Geometry check sheet. Reference: the model listing, model coordinates, mm. A direction names the side the tool comes from. Round coordinates to 2 decimals unless told otherwise and drop trailing zeros. Order: outer loops, then holes, each group sorted by start corner. A loop starts at its lowest first (then second) coordinate and runs counter-clockwise, first axis right, second up.
(1) Sectioned sample at B-B (z = -223.5). Record the boundary of the cut face in (x, y), plus the area to 3 significant figures.
(2) Material ranges on line 1 along Z through (x, y) = (-279.5, 146.5); line 2 along Y through (x, z) = (-217, -430); line 3 along Z through (x, y) = (-248.5, 277.5), recorded low to high.
(3) Release check for a two-part mould opening along Z. For faces 4 (the face through (-254, 218, -240)), 5 (the face through (-301, 225, -225)), 6 (the face through (-305.51, 182.74, -204.18)) record: +Z half, -Z half, draft (parallel to the pull), parting line (faces both ways), or undercut.
(4) Sectioned sample at C-C (x = -242). Record the boundary of the cut face in (y, z) (3 decimals).
(5) Sectioned sample at A-A (y = 182.5). Record the boundary of the cut face in (x, z).
(6) Go/stop test with flat-tipped pins: pin 1 (4 mm diameter, centred on x = -132.5, z = -308.5, fed in from -Y); pin 2 (6 mm diameter, centred on x = -491, y = 325, fed in from +Z); pin 3 (6 mm diameter, centred on x = -537.5, z = -295.5, fed in from -Y). Record where each tip stops, or that it passes through.
(7) Sectioned sample at D-D (y = 88). Record the boundary of the cut face in (x, z), plus the area to 3 significant figures.
(8) Set-up check for faces 1 (the face through (-304.089, 254.483, -276.121)), 2 (the face through (-305.511, 208.996, -248.735)), 3 (the face through (-355.6, 219, -241)): record each of +Z, -Z, +X, -X, +Y, -Y from which the full face is reachable in a straight line by a thin tool's end or side.
Autodesk Inventor part; units mm, degrees
ref_plane "YZ Plane" through (0, 0, 0) normal (1, 0, 0) x (0, 1, 0)
ref_plane "XZ Plane" through (0, 0, 0) normal (0, 1, 0) x (-1, 0, 0)
ref_plane "XY Plane" through (0, 0, 0) normal (0, 0, 1) x (1, 0, 0)
sketch "Sketch6" plane through (0, 0, 0) normal (0, 1, 0) x (-1, 0, 0)
  line L0 (0, 0) -> (609.6, 0)
  line L1 (609.6, 0) -> (609.6, -914.4)
  line L2 (609.6, -914.4) -> (0, -914.4)
  line L3 (0, -914.4) -> (0, 0)
  dimension "d21" = 609.6
  dimension "d22" = 914.4
extrude "Extrusion6" add sketch "Sketch6" along normal blind 609.6
sketch "Sketch8" plane through (0, 0, 0) normal (1, 0, 0) x (0, 0, -1)
  line L0 (0, 609.6) -> (914.4, 609.6)
  line L1 (0, 0) -> (457.2, 0) construction
  line L2 (0, 0) -> (457.2, 457.2)
  line L3 (0, 0) -> (646.5784, 0) construction
  line L4 (457.2, 457.2) -> (914.4, 0)
  line L5 (457.2, 457.2) -> (459.4451, 454.9549)
  line L6 (0, 0) -> (3.175, 0)
  line L7 (3.175, 0) -> (459.4451, 454.9549)
  dimension "d29" = 45
  dimension "d30" = 3.175
  dimension "d31" = 3.175
extrude "Extrusion7" cut sketch "Sketch8" against normal blind 609.6 keep common part
sketch "Sketch10" plane through (-609.6, 0, -3.175) normal (0, -0.7081, -0.7061) x (1, 0, 0)
  line L0 (609.6, -644.334) -> (609.6, 0)
  line L1 (609.6, 0) -> (0, 0)
  line L2 (0, 0) -> (0, -644.334)
  line L3 (609.6, -644.334) -> (0, -644.334)
  line L4 (609.6, -644.3295) -> (0, -644.3295)
  line L5 (304.8, -644.3295) -> (304.8, 2.2483)
  line L6 (609.6, 2.2483) -> (0, 2.2483)
  line L7 (609.6, -322.167) -> (0, -322.167)
  line L8 (254, -271.367) -> (355.6, -271.367)
  line L9 (355.6, -271.367) -> (355.6, -372.967)
  line L10 (355.6, -372.967) -> (254, -372.967)
  line L11 (254, -372.967) -> (254, -271.367)
  line L12 (254, -271.367) -> (355.6, -372.967) construction
  line L13 (355.6, -271.367) -> (254, -372.967) construction
  point P0 (304.8, -322.167)
  dimension "d37" = 101.6
  dimension "d38" = 101.6
extrude "Extrusion8" add sketch "Sketch10" along normal blind 25.4 contours L9 L10 L5 L7 | L7 L5 L8 L9 | L10 L11 L7 L5 | L7 L11 L8 L5
properties part number "BackV1" material "Aluminum 6061"
Answer below:
1. outline: (-609.6, 219.69) - (-355.6, 219.69) - (-355.6, 183.83) - (-254, 183.83) - (-254, 219.69) - (0, 219.69) - (0, 223.5) - (-609.6, 223.5) - close
1. area: 5,970 mm2
2. line 1: z = -150.1 to -146.5
2. line 2: y = 425.59 to 430
2. line 3: z = -281.48 to -277.5
3. face 4: draft
3. face 5: +Z half
3. face 6: undercut
4. outline: (0, -3.175) - (454.955, -459.445) - (457.2, -457.2) - (0, 0) - close
5. outline: (-609.6, -186.2) - (0, -186.2) - (0, -182.5) - (-609.6, -182.5) - close; (-355.6, -222.16) - (-254, -222.16) - (-254, -204.42) - (-355.6, -204.42) - close
6. pin 1: stops at y = 302.45
6. pin 2: stops at z = -322
6. pin 3: stops at y = 288.49
7. outline: (-609.6, -91.43) - (0, -91.43) - (0, -88) - (-609.6, -88) - close
7. area: 2,090 mm2
8. face 1: -Z, +X, -X
8. face 2: -Z, +X, -X, -Y
8. face 3: -Z, -X, -Y
